Geometry: see drawing. Coordinates: mm, zero at the bounding-box minimum. Coordinates: 2 decimals unless noted, no trailing zeros. Order: outer loops, then holes, each group sorted by start corner. A loop starts at its lowest first (then second) coordinate and runs counter-clockwise, first axis right, second up. Notation, with made-up numbers: M 24,18 L 82,18 A23 ccw 82,34 Z; hole C 32.25,71.5 d4. An arc over 180 degrees is marked long. One line per item, written item: value.
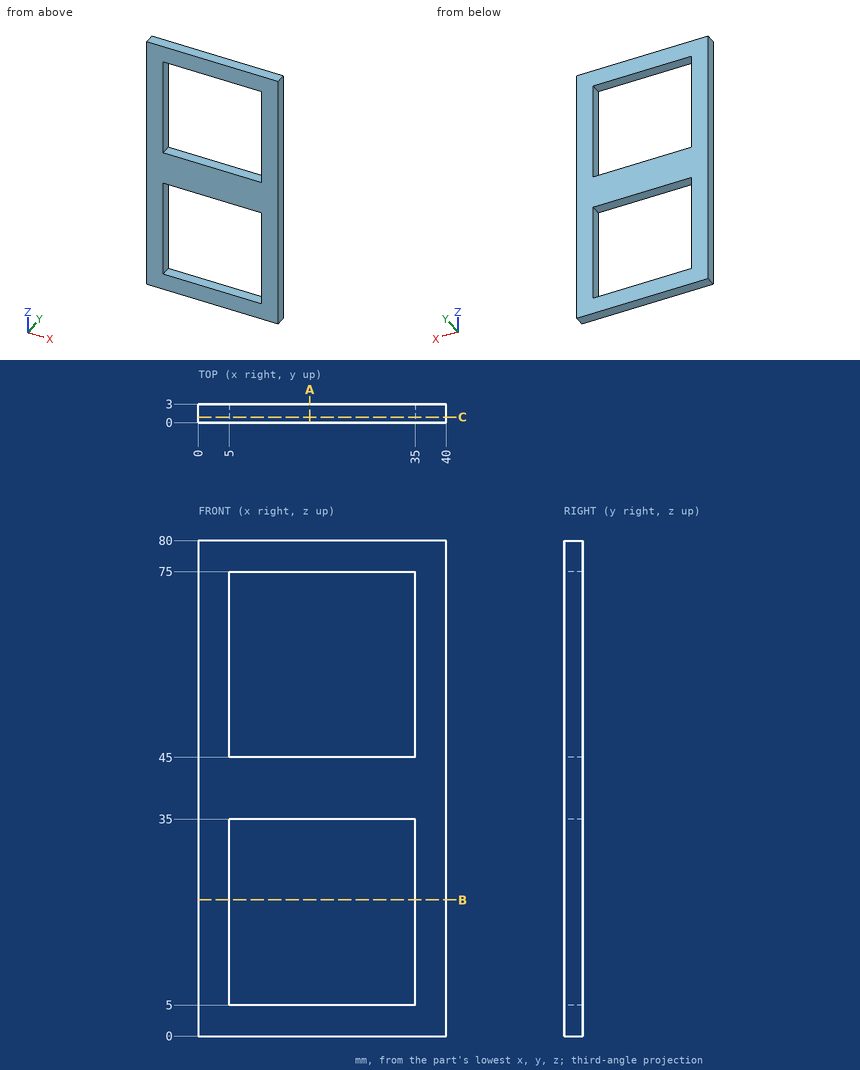
(1) Cut plane C-C on y = 0.9. Output: boundary loops of the cut face in (x, z).
Data:
outline: M 0,0 L 40,0 L 40,80 L 0,80 Z; hole M 5,5 L 35,5 L 35,35 L 5,35 Z; hole M 5,45 L 35,45 L 35,75 L 5,75 Z
(2) Ray query, line 1 (Z direction, x = 15.5, y = 0.95); line 2 (X direction, y = 0.7, z = 60). Return the intervals inside material, ascending. Write a range as from..to.
Data:
line 1: z = 0..5, 35..45, 75..80
line 2: x = 0..5, 35..40
(3) First-contact query: pin 1 (1 mm diameter, centred on x = 27.5, z = 40.5, fed in from -Y). Flat tip, straight axial feed; report the tip coordinate or a pass-through.
Data:
pin 1: stops at y = 0
(4) Cut plane A-A on x = 18. Output: boundary loops of the cut face in (y, z), plus the area to 3 significant figures.
Data:
outline: M 0,0 L 3,0 L 3,5 L 0,5 Z; M 0,35 L 3,35 L 3,45 L 0,45 Z; M 0,75 L 3,75 L 3,80 L 0,80 Z
area: 60.0 mm2
(5) Cut plane B-B on z = 22. Output: boundary loops of the cut face in (x, y).
Data:
outline: M 0,0 L 5,0 L 5,3 L 0,3 Z; M 35,0 L 40,0 L 40,3 L 35,3 Z
